from build123d import *

# Parameters (mm, degrees)
SKETCH_1_W          = 48
SKETCH_1_H          = 43
EXTRUDE_1_DEPTH     = 5
SKETCH_2_W          = 32
SKETCH_2_H          = 40
CUT_EXTRUDE_1_DEPTH = 2.5
SKETCH_3_R          = 2.1
CUT_EXTRUDE_2_DEPTH = 65.637450445
FILLET_1_R          = 2
CHAMFER_2_SIZE      = 2
SKETCH_4_W          = 32
SKETCH_4_H          = 8.9
CUT_EXTRUDE_3_DEPTH = 65.492247596


with BuildPart() as part:
    # Эскиз1 → Бобышка-Вытянуть1 (new body)
    with BuildSketch(Plane(origin=(0, 0, 0), x_dir=(1, 0, 0), z_dir=(0, 1, 0))):
        with Locations((-24, 21.5)):
            Rectangle(SKETCH_1_W, SKETCH_1_H)
    extrude(amount=-EXTRUDE_1_DEPTH)

    # Эскиз2 → Вырез-Вытянуть1 (cut)
    with BuildSketch(Plane(origin=(0, 0, 0), x_dir=(1, 0, 0), z_dir=(0, 1, 0))):
        with Locations((-24, 20)):
            Rectangle(SKETCH_2_W, SKETCH_2_H)
    extrude(amount=-CUT_EXTRUDE_1_DEPTH, mode=Mode.SUBTRACT)

    # Эскиз3 → Вырез-Вытянуть2 (cut, through all)
    with BuildSketch(Plane(origin=(0, 0, 0), x_dir=(1, 0, 0), z_dir=(0, 1, 0))):
        with Locations(Location((-44, 39, 0), (0, 0, 270))):
            Circle(SKETCH_3_R)
        with Locations(Location((-4, 39, 0), (0, 0, 90))):
            Circle(SKETCH_3_R)
        with Locations(Location((-4, 4, 0), (0, 0, 270))):
            Circle(SKETCH_3_R)
        with Locations(Location((-44, 4, 0), (0, 0, 90))):
            Circle(SKETCH_3_R)
    extrude(amount=-CUT_EXTRUDE_2_DEPTH, mode=Mode.SUBTRACT)

    # Скругление1
    fillet_1_edges = [part.edges().sort_by_distance(p)[0] for p in [
        (-48, -2.5, -43),
        (0, -2.5, -43),
        (0, -2.5, 0),
        (-48, -2.5, 0),
    ]]
    fillet(fillet_1_edges, radius=FILLET_1_R)

    # Фаска2
    chamfer_2_edges = [part.edges().sort_by_distance(p)[0] for p in [
        (-24, 0, -40),
    ]]
    chamfer(chamfer_2_edges, length=CHAMFER_2_SIZE)

    # Эскиз4 → Вырез-Вытянуть3 (cut, through all)
    with BuildSketch(Plane(origin=(0, -2.5, 0), x_dir=(1, 0, 0), z_dir=(0, 1, 0))):
        with Locations((-24, 4.45)):
            Rectangle(SKETCH_4_W, SKETCH_4_H)
    extrude(amount=-CUT_EXTRUDE_3_DEPTH, mode=Mode.SUBTRACT)


solid = part.part
Read the model definition and answer for the solid it produces. Units are mm, in the model's axes. A direction names the side the tool comes from. Round coordinates to 2 decimals unless told otherwise and drop trailing zeros. Loops run counter-clockwise (first coordinate to the right, second up) from the corner with the lowest first, then second, coordinate; pieces in that order, holes last.
Q1. Each of these flat-tipped pins is pushed along its axis until it touches: pin 1 (9.5 mm diameter, centred on x = -17.5, z = -25.5, fed in from +Y); pin 2 (4 mm diameter, centred on x = -44, z = -39, fed in from -Y); pin 3 (2 mm diameter, centred on x = -24.5, y = -3.5, fed in from +Z). Where does it stop, or does it pass through?
Q2. Which of the six approach directions +Z, -Z, +X, -X, +Y, -Y give full straight-line access (tool end or side, diameter ignored) to faces 4 (the face through (-8, -2, -16)), 5 (the face through (-24, -4, -8.9)), 6 (the face through (-43, -2, 0))?
Q3. Consider probe 1 along X at (y, z) = (-3, -39); probe 2 along X at (y, z) = (-1.4, -4); probe 3 along X at (y, z) = (-1.65, -28.5). Determine where each line is inside the solid, lowest interval first.
Q4. Section B-B on x = -4 is taken. Write down the section's boundary in (y, z), and give its area (3 significant figures).
Q5. Section A-A on z = -39 is taken. Write down the section's boundary in (x, y).
Q6. Section D-D on z = -4 is taken. Write down the section's boundary in (x, y), and give its area (3 significant figures).
Q7. Section C-C on y = -0.7 is taken. Write down the section's boundary in (x, z), and give its area (3 significant figures).
Q8. Determine the mould class of faces 1 (the face through (-24, -2, -43)), 2 (the face through (-45.278, -2.465, -40.666)), 3 (the face through (-47.43, -2.54, -42.4)) for opening direction X: released by +X, released by -X, zero draft, split by the parting line, or undercut.
Output:
1. pin 1: stops at y = -2.5
1. pin 2: passes through
1. pin 3: stops at z = -8.9
2. face 4: +Z, +Y
2. face 5: +Z, +Y, -Y
2. face 6: +Z, +X, -X, +Y, -Y
3. probe 1: x = -48 to -46.1, -41.9 to -6.1, -1.9 to 0
3. probe 2: x = -48 to -46.1, -41.9 to -40, -8 to -6.1, -1.9 to 0
3. probe 3: x = -48 to -40, -8 to 0
4. outline: (-5, -43) - (0, -43) - (0, -41.1) - (-5, -41.1) - close; (-5, -36.9) - (0, -36.9) - (0, -6.1) - (-5, -6.1) - close; (-5, -1.9) - (0, -1.9) - (0, 0) - (-5, 0) - close
4. area: 173 mm2
5. outline: (-48, -5) - (-46.1, -5) - (-46.1, 0) - (-48, 0) - close; (-41.9, -5) - (-6.1, -5) - (-6.1, 0) - (-8, 0) - (-8, -2.5) - (-40, -2.5) - (-40, 0) - (-41.9, 0) - close; (-1.9, -5) - (0, -5) - (0, 0) - (-1.9, 0) - close
6. outline: (-48, -5) - (-46.1, -5) - (-46.1, 0) - (-48, 0) - close; (-41.9, -5) - (-40, -5) - (-40, 0) - (-41.9, 0) - close; (-8, -5) - (-6.1, -5) - (-6.1, 0) - (-8, 0) - close; (-1.9, -5) - (0, -5) - (0, 0) - (-1.9, 0) - close
6. area: 38.0 mm2
7. outline: (-48, -41) arc R2 ccw to (-46, -43) - (-2, -43) arc R2 ccw to (0, -41) - (0, -2) arc R2 ccw to (-2, 0) - (-8, 0) - (-8, -41.3) - (-40, -41.3) - (-40, 0) - (-46, 0) arc R2 ccw to (-48, -2) - close; hole circle Ø4.2 at (-44, -39); hole circle Ø4.2 at (-44, -4); hole circle Ø4.2 at (-4, -39); hole circle Ø4.2 at (-4, -4)
7. area: 684 mm2
8. face 1: zero draft
8. face 2: undercut
8. face 3: released by -X
